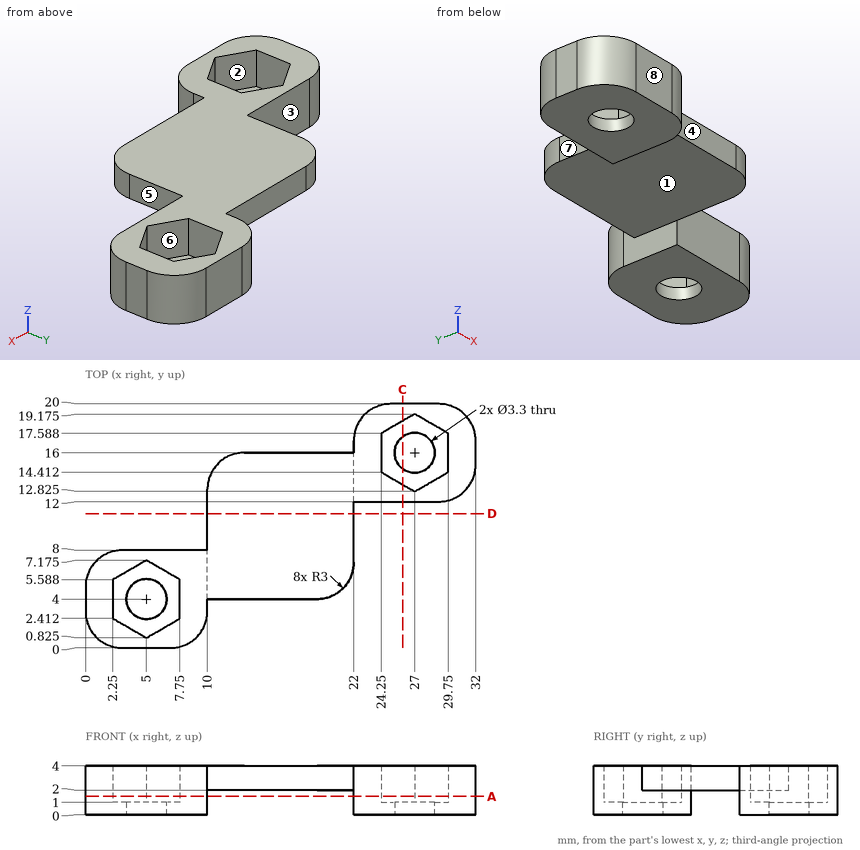
Answer from the drawing. Dimensions are ordinates in mm from the lowest x, y and z of the part. A direction names the side the tool comes from. Give positions to 0.01 mm unless a question says otherwise; leave off trailing zeros. Write each loop counter-clockwise with the first axis right and the second up, starting at its lowest first coordinate (ties: lowest second). Pieces come first, ordered by that corner, then holes. Notation, with made-up numbers: (54, -13) -> (91, -13) arc R21 cw to (91, 2) -> close; hole circle Ø3 at (33.5, 20.5). An arc over 180 degrees is marked (long way). One line per question, with ' | ' between items. Start each with the question number.
1. For the marked faces 1, 2, 3 and 4, determine the directions among +Z, -Z, +X, -X, +Y, -Y from which every point of the face is accessible in a straight line to the end or side of a thin tool.
2. Section D-D (y = 11) is taken. Determine the outline of the cut face in (x, z), plus the area to 3 significant figures.
3. Find the intervals of material crossed by probe 1 along X at (y, z) = (16, 0.6); probe 2 along Y at (x, z) = (27, 0.6); probe 3 along X at (y, z) = (4, 0.35), in increasing order.
4. Section C-C (x = 26) is taken. Determine the outline of the cut face in (y, z), plus the area to 3 significant figures.
5. Given pin 1 Ø2 at (y, z) = (4.5, 1.5) entering from +X (1 decimal); pin 2 Ø2 at (y, z) = (9.5, 3) entering from +X; pin 3 Ø6 at (x, y) = (22.5, 3.5) entering from -Z; pin 4 Ø2 at (x, y) = (5, 4) entering from -Z, each flat-ended and moving along its own axis, determine where each tip first touches the part or whether it passes through.
6. For a pull along X with two mould halves and no side action, classify the marked faces 5, 6, 7 and 8 as pulls with the +X half, pulls with the -X half, needs draft (parallel to the pull), parting line crosses it, or undercut.
7. Section A-A (z = 1.5) is taken. State how many separate pieces and enclosed holes the cut face has.
Response values:
1) face 1: -Z, +Y, -Y | face 2: +Z | face 3: +Z, -Z, -X, +Y | face 4: +Z, -Z, +X, -Y
2) outline: (10, 2) -> (22, 2) -> (22, 4) -> (10, 4) -> close | area: 24.0 mm2
3) probe 1: 22 to 25.35, 28.65 to 32 | probe 2: 12 to 14.35, 17.65 to 20 | probe 3: 0 to 3.35, 6.65 to 10
4) outline: (12, 0) -> (14.69, 0) -> (14.69, 1) -> (13.4, 1) -> (13.4, 4) -> (12, 4) -> close; (17.31, 0) -> (20, 0) -> (20, 4) -> (18.6, 4) -> (18.6, 1) -> (17.31, 1) -> close | area: 13.8 mm2
5) pin 1: x = 21.5 | pin 2: x = 22 | pin 3: z = 2 | pin 4: through
6) face 5: pulls with the +X half | face 6: undercut | face 7: pulls with the -X half | face 8: needs draft
7) separate pieces: 2 | enclosed holes: 2
